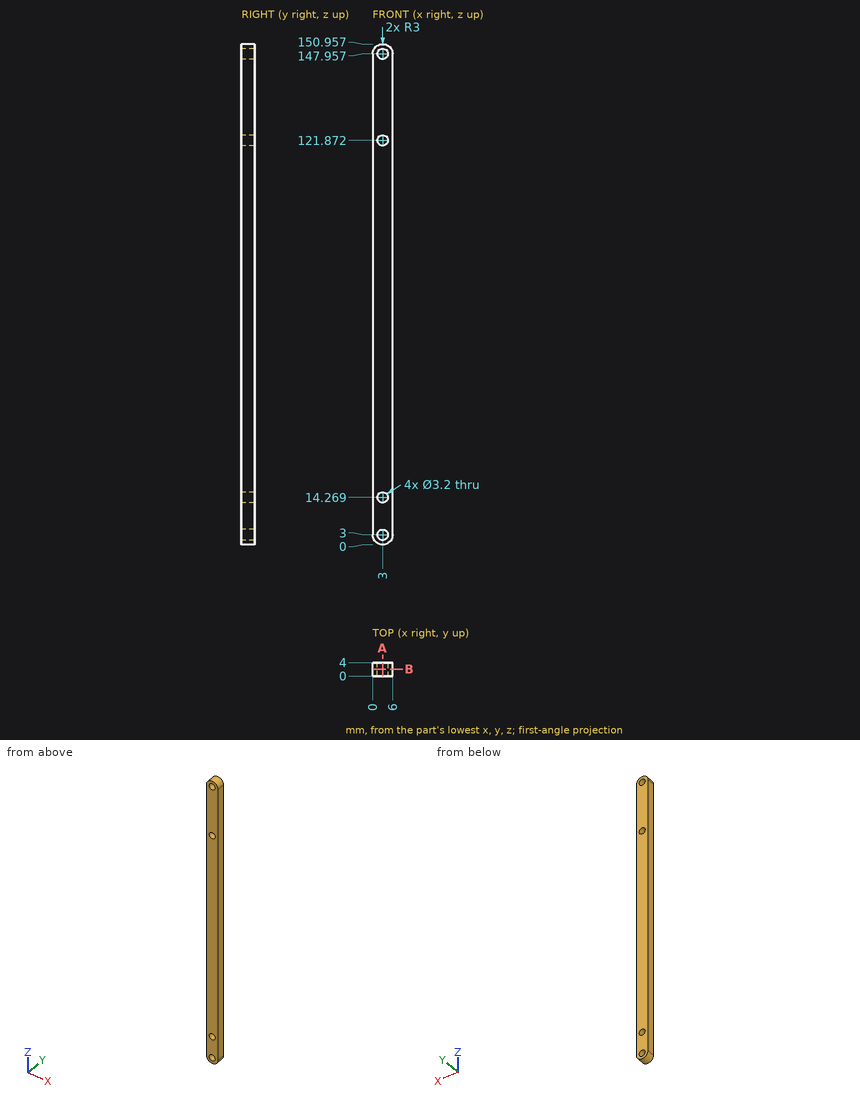
Input: dimensioned drawing with shaded views. Units: mm. Origin: part minimum x, y, z. Coordinates: 2 decimals unless noted, no trailing zeros. Loops run counter-clockwise (first coordinate to the right, second up) from the corner with the lowest first, then second, coordinate; pieces in that order, holes last. Notation, with made-up numbers: (13.25, 33.25) -> (27.25, 33.25) arc R27 ccw to (27.25, 65.25) -> close; hole circle Ø1 at (63, 29.25). An arc over 180 degrees is marked (long way). Use a Markdown table: item, result. Add a question column.
(1) Line query: line 1 along Z through (x, y) = (2.9, 0.6); line 2 along Z through (x, y) = (2.8, 2.2); line 3 along Z through (x, y) = (5.55, 1.75). Output: solid intervals per line, ascending.
(2) Section query B-B, the plane y = 2.1. Return loops of the section in (x, z), plus the area to 3 significant figures.
(3) Section query A-A, the plane x = 3. Return loops of the section in (y, z).
(4) Pin query (flat end, axial travel): pin 1 Ø2.5 at (x, z) = (3, 14.269) entering from +Y. Return the tip coordinate at first contact, or that it passes through.
Answer:
| question | item | result |
|---|---|---|
| 1 | line 1 | z = 0 to 1.4, 4.6 to 12.67, 15.87 to 120.28, 123.47 to 146.36, 149.55 to 150.96 |
| 1 | line 2 | z = 0.01 to 1.41, 4.59 to 12.68, 15.86 to 120.28, 123.46 to 146.37, 149.54 to 150.95 |
| 1 | line 3 | z = 1.42 to 149.54 |
| 2 | outline | (0, 3) arc R3 ccw to (6, 3) -> (6, 147.96) arc R3 ccw to (0, 147.96) -> close; hole circle Ø3.2 at (3, 3); hole circle Ø3.2 at (3, 14.27); hole circle Ø3.2 at (3, 121.87); hole circle Ø3.2 at (3, 147.96) |
| 2 | area | 866 mm^2 |
| 3 | outline | (0, 0) -> (4, 0) -> (4, 1.4) -> (0, 1.4) -> close; (0, 4.6) -> (4, 4.6) -> (4, 12.67) -> (0, 12.67) -> close; (0, 15.87) -> (4, 15.87) -> (4, 120.27) -> (0, 120.27) -> close; (0, 123.47) -> (4, 123.47) -> (4, 146.36) -> (0, 146.36) -> close; (0, 149.56) -> (4, 149.56) -> (4, 150.96) -> (0, 150.96) -> close |
| 4 | pin 1 | passes through |
